Geometry check sheet. Reference: the model listing, model coordinates, mm. A direction names the side the tool comes from. Round coordinates to 2 decimals unless told otherwise and drop trailing zeros. Order: outer loops, then holes, each group sorted by start corner. A loop starts at its lowest first (then second) coordinate and runs counter-clockwise, first axis right, second up. Notation, with made-up numbers: (-18, 84.5) - (40, 84.5) arc R18 ccw to (40, 91.5) - close; hole circle Ø6 at (-20.5, 64). An arc over 180 degrees is marked (long way). Return JSON: item names as keys, results as strings. Group by question number.
Q1. Sectioned sample at B-B, the plane y = 0. Record the cut outline in (x, z).
Q2. Sectioned sample at A-A, the plane x = 0. Record the cut outline in (y, z), then the cut area to 3 significant figures.
Q3. Material ranges on line 1 along Y through (x, z) = (0, 16); line 2 along Y through (x, z) = (0, 5.5), recorded low to high.
Q4. Gauge pin test, flat ends, axial feed: pin 1 Ø4 at (x, z) = (-2.5, 10) entering from -Y; pin 2 Ø4 at (x, z) = (0.5, 15) entering from +Y; pin 3 Ø1.5 at (y, z) = (1.5, 13.5) entering from +X. Record the tip position at first contact, or that the pin passes through.
Q5. Tool access check on faces 1 (the cylindrical face through (0, -2, 18)), 2 (the cylindrical face through (2.86, 0.9, 0.13)), 3 (the flat face through (1, -1, 20)). Record the directions out of +Z, -Z, +X, -X, +Y, -Y that give a thin tool (end or side, any length) a straight path to the whole face; none if there is none.
Q6. Sectioned sample at D-D, the plane z = 16.5. Record the cut outline in (x, y), then the cut area to 3 significant figures.
Q7. Sectioned sample at C-C, the plane z = 2. Record the cut outline in (x, y).
```python
from build123d import *

# Parameters (mm, degrees)
SKETCH005_R      = 1.2
EXTRUDE005_DEPTH = 30
SKETCH003_R      = 8
EXTRUDE004_DEPTH = 10
SKETCH002_R      = 3
EXTRUDE003_DEPTH = 12
SKETCH001_R      = 9.2
EXTRUDE001_DEPTH = 10
SKETCH_R         = 4
EXTRUDE_DEPTH    = 10


with BuildPart() as extrude005:
    # Sketch005 → Extrude005 (new body)
    with BuildSketch(Plane.XY.offset(20)):
        Circle(SKETCH005_R)
    extrude(amount=-EXTRUDE005_DEPTH)


with BuildPart() as extrude004:
    # Sketch003 → Extrude004 (new body, symmetric)
    with BuildSketch(Plane.XZ):
        with Locations((0, -8.2)):
            Circle(SKETCH003_R)
    extrude(amount=EXTRUDE004_DEPTH, both=True)


with BuildPart() as cut001:
    # Sketch002 (on Face3 of Cut) → Extrude003 (new body)
    with BuildSketch(Plane.XY.offset(10)):
        Circle(SKETCH002_R)
    extrude(amount=-EXTRUDE003_DEPTH)

    # Cut001: cut Extrude004
    add(extrude004.part, mode=Mode.SUBTRACT)


with BuildPart() as extrude001:
    # Sketch001 → Extrude001 (new body, symmetric)
    with BuildSketch(Plane.XZ):
        with Locations((0, -8.2)):
            Circle(SKETCH001_R)
    extrude(amount=EXTRUDE001_DEPTH, both=True)


with BuildPart() as cut004:
    # Sketch → Extrude (new body)
    with BuildSketch(Plane.XY):
        Circle(SKETCH_R)
    extrude(amount=EXTRUDE_DEPTH)

    # Cut: cut Extrude001
    add(extrude001.part, mode=Mode.SUBTRACT)

    # Fusion: union Cut001
    add(cut001.part)

    # Cut003: cut Extrude005
    add(extrude005.part, mode=Mode.SUBTRACT)

    # Cut004: cut Extrude005
    add(extrude005.part, mode=Mode.SUBTRACT)


with BuildPart() as fusion001:
    # Sketch004 → Revolve (revolve)
    with BuildSketch(Plane.XZ):
        Polygon((1.2, 10), (4, 10), (2, 15.494955), (2, 20), (1.2, 20), align=None)
    revolve(axis=Axis((0, 0, 0), (0, 0, 1)))

    # Fusion001: union Cut004
    add(cut004.part)


solid = fusion001.part
```
Reply:
{
 "1": {"outline": "(-4, 0.08) arc R9.2 cw to (-3, 0.5) - (-3, -0.78) arc R8 cw to (-1.2, -0.29) - (-1.2, 20) - (-2, 20) - (-2, 15.49) - (-4, 10) - close; (1.2, -0.29) arc R8 cw to (3, -0.78) - (3, 0.5) arc R9.2 cw to (4, 0.08) - (4, 10) - (2, 15.49) - (2, 20) - (1.2, 20) - close"},
 "2": {"outline": "(-4, 1) - (-3, 1) - (-3, -0.2) - (-1.2, -0.2) - (-1.2, 20) - (-2, 20) - (-2, 15.49) - (-4, 10) - close; (1.2, -0.2) - (3, -0.2) - (3, 1) - (4, 1) - (4, 10) - (2, 15.49) - (2, 20) - (1.2, 20) - close", "area": "81.7 mm^2"},
 "3": {"line 1": "-2 to -1.2, 1.2 to 2", "line 2": "-4 to -1.2, 1.2 to 4"},
 "4": {"pin 1": "y = -3.97", "pin 2": "y = 2.89", "pin 3": "x = 2.75"},
 "5": {"face 1": "+Z", "face 2": "-Z", "face 3": "+Z, +X, -X, +Y, -Y"},
 "6": {"outline": "circle Ø4 at (0, 0); hole circle Ø2.4 at (0, 0)", "area": "8.04 mm^2"},
 "7": {"outline": "circle Ø8 at (0, 0); hole circle Ø2.4 at (0, 0)"}
}
